from build123d import *

# Parameters (mm, degrees)
F0_W     = 539.75
F0_H     = 20.6375
F1_DEPTH = 260.35
F2_W     = 11.1125
F2_H     = 11.1125
F3_DEPTH = 260.351
F4_W     = 517.525
F4_H     = 22.225
F5_DEPTH = 11.1125


with BuildPart() as f1:
    # F0 (on Top) → F1 (new body)
    with BuildSketch(Plane.XY):
        with Locations((0, 10.31875)):
            Rectangle(F0_W, F0_H)
    extrude(amount=-F1_DEPTH)

    # F2 (on face) → F3 (cut, through all)
    with BuildSketch(Plane.XY):
        with Locations((-264.31875, 15.08125)):
            Rectangle(F2_W, F2_H)
        with Locations((264.31875, 15.08125)):
            Rectangle(F2_W, F2_H)
    extrude(amount=-F3_DEPTH, mode=Mode.SUBTRACT)

    # F4 (on face) → F5 (cut, through all)
    with BuildSketch(Plane(origin=(0, 20.6375, 0), x_dir=(-1, 0, 0), z_dir=(0, 1, 0))):
        with Locations((0, -20.6375)):
            Rectangle(F4_W, F4_H)
    extrude(amount=-F5_DEPTH, mode=Mode.SUBTRACT)


solid = f1.part
Can you work these out from the model? Positions are in its coordinate system, mm. A direction names the side the tool comes from. Give positions to 0.01 mm unless a question says otherwise; leave off trailing zeros. Order: outer loops, then holes, each group sorted by start corner. A loop starts at its lowest first (then second) coordinate and runs counter-clockwise, first axis right, second up. Notation, with made-up numbers: M 55,16 L 67,16 A19 cw 67,50 Z; hole C -31,-32 d5. An arc over 180 degrees is marked long. Use a Markdown table: item, result. Add a question column.
Item 1: Suppose I cut it at D-D (z = -21). List the corners of the cut face in (x, y) for me (3 decimals).
Item 2: If I drill on L1, parallel to Z at x = 150.5, y = 9.75 (3 decimals); L2, parallel to X at y = 15.75, z = -123, over which ranges is the centre line in solid material (lowest first)? Write a range as [from, to].
Item 3: For faces 1 (the flat face through (4, 15, -9.525)), 2 (the flat face through (-269.875, 5, -128)), 3 (the flat face through (-4, 0, -128)), 4 (the flat face through (-258.763, 15, -144)), 5 (the flat face through (258.763, 15, -144)), which set-ups out of +Z, -Z, +X, -X, +Y, -Y let a thin tool reach every point of the face, with its end or its side?
Item 4: Will these pins go through, and if not, where does the flat tip stop? pin 1 (3.5 mm diameter, centred on y = 14.5, z = -123, fed in from -X); pin 2 (9 mm diameter, centred on y = 17.5, z = -165.5, fed in from +X).
Item 5: We'd pull the mould along Z, two halves only. Please class faces 6 (the flat face through (-81, 9.525, -23)), 7 (the flat face through (-4, 10, -260.35)), 8 (the flat face through (-258.763, 15, -5)): +Z half, -Z half, draft (parallel to the pull), parting line (faces both ways), or undercut.
Item 6: Suppose I cut it at C-C (z = -60.5). List the corners of the cut face in (x, y) for me (1 decimal).
Answer sheet:
| question | item | result |
|---|---|---|
| 1 | outline | M -269.875,0 L 269.875,0 L 269.875,9.525 L -269.875,9.525 Z |
| 2 | L1 | z = [-260.35, -31.75], [-9.525, 0] |
| 2 | L2 | x = [-258.76, 258.76] |
| 3 | face 1 | +X, -X, +Y |
| 3 | face 2 | +Z, -Z, -X, +Y, -Y |
| 3 | face 3 | +Z, -Z, +X, -X, -Y |
| 3 | face 4 | +Z, -Z, -X, +Y |
| 3 | face 5 | +Z, -Z, +X, +Y |
| 4 | pin 1 | stops at x = -258.76 |
| 4 | pin 2 | stops at x = 258.76 |
| 5 | face 6 | undercut |
| 5 | face 7 | -Z half |
| 5 | face 8 | draft |
| 6 | outline | M -269.9,0 L 269.9,0 L 269.9,9.5 L 258.8,9.5 L 258.8,20.6 L -258.8,20.6 L -258.8,9.5 L -269.9,9.5 Z |
